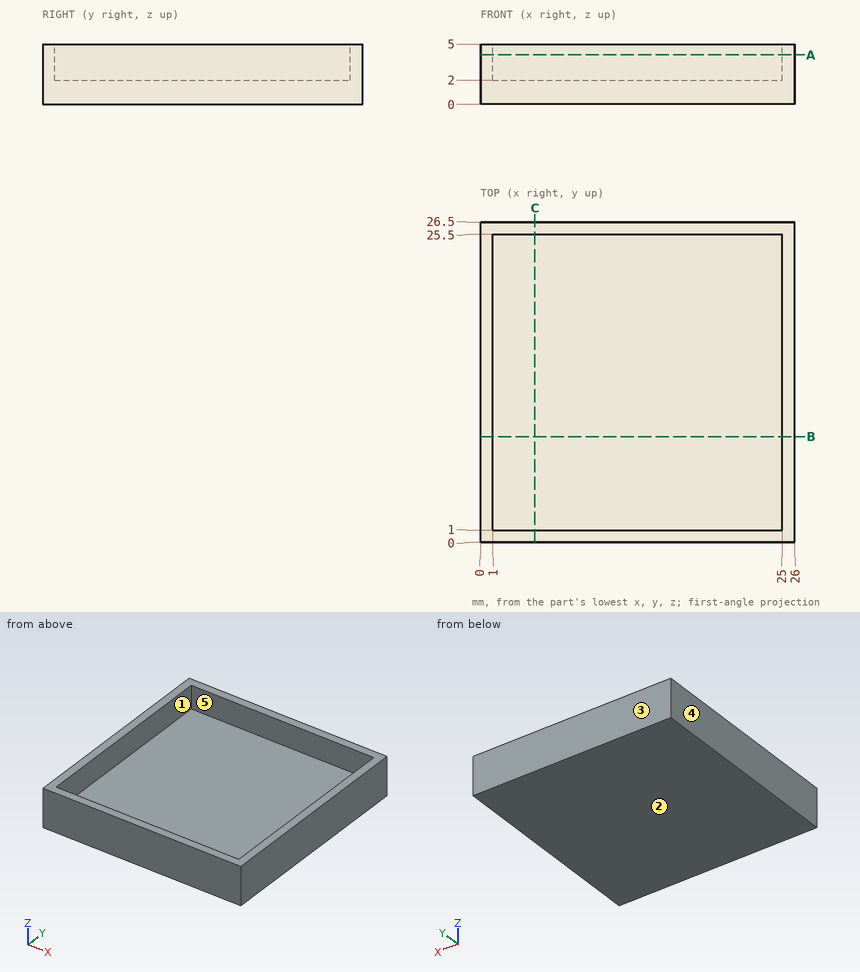
Design review of the part shown in the three views and the two pictorial views. Dimensions are in mm from the part's minimum x, y and z. A direction names the side the tool comes from. Coordinates: 2 decimals unless noted, no trailing zeros. Write each loop counter-clockwise with the first axis right and the second up, starting at its lowest first coordinate (ties: lowest second). Pieces come first, ordered by that corner, then holes.
1) The part is to be moulded in two halves that separate along Y. For the marked faces 3, 4 and 5, say which applies: pulls with the +Y half, pulls with the -Y half, needs draft (parallel to the pull), parting line crosses it, or undercut.
2) To check wall thickness, follow probe 1 along X at (y, z) = (16, 4.7); probe 2 along Y at (x, z) = (17.25, 2.45); probe 3 along Z at (x, y) = (7, 5.5). State the ranges of each line that lie inside material, in increasing order.
3) We need section B-B on y = 8.75. State the section outline as (x, z) points.
4) We need section C-C on x = 4.5. State the section outline as (y, z) points.
5) Clearance check with flat-ended pins moving along their axes: pin 1 Ø7 at (x, y) = (12.5, 10.5) entering from +Z; pin 2 Ø5 at (x, y) = (8, 5) entering from -Z. State where each tip first meets the part, or that it passes through.
6) Machinability: for the marked faces 1 and 2, which of the approach directions +Z, -Z, +X, -X, +Y, -Y give a long, thin tool a straight path to every point of the face, cutting with its end or side? Answer none if there is none.
7) We need section A-A on z = 4.1. State the section outline as (x, y) points.
Answer list:
1. face 3: pulls with the +Y half
1. face 4: needs draft
1. face 5: undercut
2. probe 1: x = 0 to 1, 25 to 26
2. probe 2: y = 0 to 1, 25.5 to 26.5
2. probe 3: z = 0 to 2
3. outline: (0, 0) - (26, 0) - (26, 5) - (25, 5) - (25, 2) - (1, 2) - (1, 5) - (0, 5) - close
4. outline: (0, 0) - (26.5, 0) - (26.5, 5) - (25.5, 5) - (25.5, 2) - (1, 2) - (1, 5) - (0, 5) - close
5. pin 1: stops at z = 2
5. pin 2: stops at z = 0
6. face 1: +Z
6. face 2: -Z, +X, -X, +Y, -Y
7. outline: (0, 0) - (26, 0) - (26, 26.5) - (0, 26.5) - close; hole (1, 1) - (25, 1) - (25, 25.5) - (1, 25.5) - close
